Read the model definition and answer for the solid it produces. Units are mm, in the model's axes. Round coordinates to 2 decimals unless told otherwise and drop trailing zeros. Use a Markdown table: item, result. Add a question column.
1. Given pin 1 (1.5 mm diameter, centred on x = 5, z = 68, fed in from +Y); pin 2 (8 mm diameter, centred on y = 12.5, z = 26, fed in from +X); pin 3 (1 mm diameter, centred on x = -9.5, z = 15, fed in from -Y), each flat-ended and moving along its own axis, determine where each tip first touches the part or whether it passes through.
2. The mould has two halves that part along Z. Classify faces 1 (the face through (1, 0, 0)), 2 (the face through (1, 0, 2)), 3 (the face through (8, 6, 100)): +Z half, -Z half, draft (parallel to the pull), parting line (faces both ways), or undercut.
3. Consider L1, parallel to X at y = 7.5, z = 77.5; L2, parallel to Y at x = 1, z = 70.5; L3, parallel to X at y = 6, z = 35 (3 decimals). Determine where each line is inside the solid, lowest interval first. Write a range as [from, to].
```python
from build123d import *

# Parameters (mm, degrees)
F0_W = 56.13058
F0_H = 56.130584
F4_T = -2


with BuildPart() as f3:
    # F2 (on offset) → F3 section 0
    with BuildSketch(Plane.XY.offset(100)):
        Polygon((17.008768, -0.472353), (0.110915, 16.4255), (-16.314585, 0), (0.583268, -16.897853), align=None)
    # F0 (on Top) → F3 section 1
    with BuildSketch(Plane.XY):
        Rectangle(F0_W, F0_H)
    loft()

    # F4
    f4_openings = [f3.faces().sort_by_distance(p)[0] for p in [
        (0.347092, -0.236176, 100),
    ]]
    offset(amount=F4_T, openings=f4_openings)


solid = f3.part
```
Verdict:
| question | item | result |
|---|---|---|
| 1 | pin 1 | stops at y = 18.88 |
| 1 | pin 2 | stops at x = 22.99 |
| 1 | pin 3 | stops at y = -25.77 |
| 2 | face 1 | -Z half |
| 2 | face 2 | undercut |
| 2 | face 3 | +Z half |
| 3 | L1 | x = [-16.6, -12.03], [10, 12.28] |
| 3 | L2 | y = [-16.54, -14.37], [14.66, 16.83] |
| 3 | L3 | x = [-22.245, -20.205], [18.731, 20.791] |
